```python
from build123d import *

# Parameters (mm, degrees)
SKETCH1_R                            = 6
BOSS_EXTRUDE1_DEPTH                  = 30
FILLET2_RADIUS                       = 15
FILLET2_LENGTH                       = 9
FILLET3_RADIUS                       = 15
FILLET3_LENGTH                       = 9
CUT_EXTRUDE1_DEPTH                   = 10
CUT_EXTRUDE1_DEPTH_BACK              = 59
SKETCH2_W                            = 12
SKETCH2_H                            = 40.970774173
F_12_0MM_DOWEL_HOLE1_D               = 12
F_12_0MM_DOWEL_HOLE1_DEPTH           = 10
F_12_0MM_DOWEL_HOLE1_TIP             = 3.605163714
F_12_0MM_DOWEL_HOLE1_ON_FACE_2_D     = 12
F_12_0MM_DOWEL_HOLE1_ON_FACE_2_DEPTH = 10
F_12_0MM_DOWEL_HOLE1_ON_FACE_2_TIP   = 3.605163714
FILLET4_R                            = 2


with BuildPart() as part:
    # Sketch1 → Boss-Extrude1 (new body)
    with BuildSketch(Plane.XY):
        with BuildLine():
            Line((15, 15), (15, 0))
            Line((15, 0), (45, 0))
            Line((45, 0), (45, -9))
            Line((45, -9), (7.15528467, -9))
            Line((7.15528467, -9), (-6, -9))
            Line((-6, -9), (-6, -45))
            Line((-6, -45), (-15, -45))
            Line((-15, -45), (-15, 15))
            ThreePointArc((-15, 15), (0, 30), (15, 15))
        make_face()
        with Locations((0, 15)):
            Circle(SKETCH1_R, mode=Mode.SUBTRACT)
    extrude(amount=BOSS_EXTRUDE1_DEPTH)

    # Fillet2: full round fillet: the end face becomes a half cylinder, R = half its width
    fillet2_face = Plane((45, -4.5, 15), x_dir=(0, 1, 0), z_dir=(1, 0, 0))  # on the end face: x along it, z out of the body
    fillet2_slab = fillet2_face.offset(-FILLET2_RADIUS / 2) * Box(FILLET2_LENGTH, 2 * FILLET2_RADIUS, FILLET2_RADIUS, mode=Mode.PRIVATE)  # the body's end, R deep
    fillet2_round = Plane((30, -4.5, 15), x_dir=(1, 0, 0), z_dir=(0, 1, 0)) * Cylinder(FILLET2_RADIUS, FILLET2_LENGTH, mode=Mode.PRIVATE)  # its axis R under the face
    add(fillet2_slab - fillet2_round, mode=Mode.SUBTRACT)

    # Fillet3: full round fillet: the end face becomes a half cylinder, R = half its width
    fillet3_face = Plane((-10.5, -45, 15), x_dir=(1, 0, 0), z_dir=(0, -1, 0))  # on the end face: x along it, z out of the body
    fillet3_slab = fillet3_face.offset(-FILLET3_RADIUS / 2) * Box(FILLET3_LENGTH, 2 * FILLET3_RADIUS, FILLET3_RADIUS, mode=Mode.PRIVATE)  # the body's end, R deep
    fillet3_round = Plane((-10.5, -30, 15), x_dir=(0, -1, 0), z_dir=(1, 0, 0)) * Cylinder(FILLET3_RADIUS, FILLET3_LENGTH, mode=Mode.PRIVATE)  # its axis R under the face
    add(fillet3_slab - fillet3_round, mode=Mode.SUBTRACT)

    # Sketch2 → Cut-Extrude1 (cut, two sides: drawn at the far end of the back side and taken through both)
    with BuildSketch(Plane(origin=(15, 0, 0), x_dir=(0, 0, -1), z_dir=(1, 0, 0)).offset(-CUT_EXTRUDE1_DEPTH_BACK)):
        with Locations((-15.359950539, 20.485387087)):
            Rectangle(SKETCH2_W, SKETCH2_H)
    extrude(amount=CUT_EXTRUDE1_DEPTH + CUT_EXTRUDE1_DEPTH_BACK, mode=Mode.SUBTRACT)

    # Ø12.0mm Dowel Hole1
    with Locations(Plane(origin=(30, 0, 15), x_dir=(1, 0, 0), z_dir=(0, 1, 0))):
        with Locations((0, 0)):
            Hole(F_12_0MM_DOWEL_HOLE1_D / 2, depth=F_12_0MM_DOWEL_HOLE1_DEPTH)
            with Locations((0, 0, -(F_12_0MM_DOWEL_HOLE1_DEPTH + F_12_0MM_DOWEL_HOLE1_TIP / 2))):  # 118° drill point
                Cone(0, F_12_0MM_DOWEL_HOLE1_D / 2, F_12_0MM_DOWEL_HOLE1_TIP, mode=Mode.SUBTRACT)

    # Ø12.0mm Dowel Hole1 on face 2
    with Locations(Plane(origin=(-6, -30, 15), x_dir=(0, 0, 1), z_dir=(1, 0, 0))):
        with Locations((0, 0)):
            Hole(F_12_0MM_DOWEL_HOLE1_ON_FACE_2_D / 2, depth=F_12_0MM_DOWEL_HOLE1_ON_FACE_2_DEPTH)
            with Locations((0, 0, -(F_12_0MM_DOWEL_HOLE1_ON_FACE_2_DEPTH + F_12_0MM_DOWEL_HOLE1_ON_FACE_2_TIP / 2))):  # 118° drill point
                Cone(0, F_12_0MM_DOWEL_HOLE1_ON_FACE_2_D / 2, F_12_0MM_DOWEL_HOLE1_ON_FACE_2_TIP, mode=Mode.SUBTRACT)

    # Fillet4
    fillet4_edges = [part.edges().sort_by_distance(p)[0] for p in [
        (15, 0, 25.67997527),
        (-6, -9, 15),
        (15, 0, 4.67997527),
        (0, 0, 21.359950539),
        (0, 0, 9.359950539),
    ]]
    fillet(fillet4_edges, radius=FILLET4_R)


solid = part.part
```
The listing builds one solid part. Answer for the finished solid, in the listing's coordinates (mm). A direction names the side the tool comes from. Coordinates: 2 decimals unless noted, no trailing zeros. Write each loop counter-clockwise with the first axis right and the second up, starting at its lowest first coordinate (ties: lowest second). Pieces come first, ordered by that corner, then holes. Notation, with made-up numbers: M 55.25,33 L 84.25,33 A24 ccw 84.25,52 Z; hole C 15.5,60 d4. An arc over 180 degrees is marked long. Use a Markdown table: item, result. Add a question column.
1. Section B-B (x = 0) is taken. Give the vertices of the cut face in (y, z), plus the area to 3 significant figures.
2. Section C-C (z = 27) is taken. Give the vertices of the cut face in (x, y).
3. Straight lines are drawn through the part: line 1 along Z through (x, y) = (-9, -30); line 2 along Y through (x, z) = (0, 26.25); line 3 along Y through (x, z) = (-10, 15). For each, find the intervals that lie inside material, in ascending order. Write a range as [from, to].
4. Which of the six approach directions +Z, -Z, +X, -X, +Y, -Y give full straight-line access (tool end or side, diameter ignored) to faces 1 (the cylindrical face through (1.22, 0.57, 9.96)), 2 (the flat face through (-6, -24, 18)), 3 (the flat face through (15, 9, 5))?
5. Section D-D (z = 15) is taken. Give the vertices of the cut face in (x, y), plus the area to 3 significant figures.
6. Section A-A (y = 5) is taken. Give the vertices of the cut face in (x, z).
7. Given P1, Ø2.5, axis at y = 7.5, z = 26.5, coming from the +X side; P2, Ø6, axis at x = 13.5, z = 9, coming from the +Y side; P3, Ø9, axis at x = 5.5, z = 8, coming from the +Y side; P4, Ø14, axis at x = -2, y = 16, coming from the +Z side, each flat-ended and moving along its own axis, determine where each tip first touches the part or whether it passes through.
8. For a pull along Z with two mould halves and no side action, classify faces 4 (the cylindrical face through (45, -4, 15)), 5 (the cylindrical face through (15.57, 0.6, 4.5)), 6 (the cylindrical face through (34.42, -4.56, 10.94)) as +Z half, -Z half, draft (parallel to the pull), parting line (faces both ways), or undercut.
Data:
| question | item | result |
|---|---|---|
| 1 | outline | M -9,0 L 9,0 L 9,9.36 L 2,9.36 A2 cw 0,11.36 L 0,19.36 A2 cw 2,21.36 L 9,21.36 L 9,30 L -9,30 Z; M 21,0 L 30,0 L 30,9.36 L 21,9.36 Z; M 21,21.36 L 30,21.36 L 30,30 L 21,30 Z |
| 1 | area | 596 mm2 |
| 2 | outline | M -15,-39 L -6,-39 L -6,-11 A2 cw -4,-9 L 39,-9 L 39,0 L 17,0 A2 cw 15,2 L 15,15 A15 ccw -15,15 Z; hole C 0,15 d12 |
| 3 | line 1 | z = [0, 9], [21, 30] |
| 3 | line 2 | y = [-9, 9], [21, 30] |
| 3 | line 3 | y = [-45, -36], [-24, 0] |
| 4 | face 1 | +X, -X, +Y |
| 4 | face 2 | +Z, -Z, +X, -Y |
| 4 | face 3 | +Z, -Z, +X, +Y |
| 5 | outline | M -15,-45 L -6,-45 L -6,-36 L -15,-36 Z; M -15,-24 L -6,-24 L -6,-11 A2 cw -4,-9 L 24,-9 L 24,0 L -15,0 Z; M 36,-9 L 45,-9 L 45,0 L 36,0 Z |
| 5 | area | 649 mm2 |
| 6 | outline | M -15,0 L 15,0 L 15,9.36 L -15,9.36 Z; M -15,21.36 L 15,21.36 L 15,30 L -15,30 Z |
| 7 | P1 | stops at x = 15 |
| 7 | P2 | stops at y = 25.71 |
| 7 | P3 | stops at y = 29.97 |
| 7 | P4 | stops at z = 30 |
| 8 | face 4 | parting line |
| 8 | face 5 | draft |
| 8 | face 6 | undercut |
